```python
from build123d import *

# Parameters (mm, degrees)
ESQUISSE3_R             = 2.5
BOSS_EXTRU_3_DEPTH      = 5
ESQUISSE4_W             = 40
ESQUISSE4_H             = 30
ENL_V_MAT_EXTRU_1_DEPTH = 161.669919512


with BuildPart() as part:
    # Esquisse3 → Boss.-Extru.3 (new body)
    with BuildSketch(Plane(origin=(0, 0, 0), x_dir=(1, 0, 0), z_dir=(0, 1, 0))):
        with BuildLine():
            Line((-115, -25), (-25, -25))
            Line((-25, -25), (-24.99494949, -24.500051021))
            ThreePointArc((-24.99494949, -24.500051021), (-17.805293657, -30.132565736), (-9.403186381, -33.713203436))
            Line((-9.403186381, -33.713203436), (35.849364905, -112.092921435))
            Line((35.849364905, -112.092921435), (79.150635095, -87.092921435))
            Line((79.150635095, -87.092921435), (34.150635095, -9.150635095))
            Line((34.150635095, -9.150635095), (33.715141323, -9.396235714))
            ThreePointArc((33.715141323, -9.396235714), (34.998214236, -0.353553761), (33.898083809, 8.713203436))
            Line((33.898083809, 8.713203436), (79.150635095, 87.092921435))
            Line((79.150635095, 87.092921435), (35.849364905, 112.092921435))
            Line((35.849364905, 112.092921435), (-9.150635095, 34.150635095))
            Line((-9.150635095, 34.150635095), (-8.720191833, 33.896286735))
            ThreePointArc((-8.720191833, 33.896286735), (-17.19292058, 30.486119496), (-24.494897428, 25))
            Line((-24.494897428, 25), (-115, 25))
            Line((-115, 25), (-115, -25))
        make_face()
        with Locations(Location((-110, -20, 0), (0, 0, 270))):
            Circle(ESQUISSE3_R, mode=Mode.SUBTRACT)
        with Locations(Location((-110, 20, 0), (0, 0, 270))):
            Circle(ESQUISSE3_R, mode=Mode.SUBTRACT)
        with Locations(Location((72.320508076, -85.262794416, 0), (0, 0, 270))):
            Circle(ESQUISSE3_R, mode=Mode.SUBTRACT)
        with Locations(Location((37.679491924, -105.262794416, 0), (0, 0, 270))):
            Circle(ESQUISSE3_R, mode=Mode.SUBTRACT)
        with Locations(Location((72.320508076, 85.262794416, 0), (0, 0, 270))):
            Circle(ESQUISSE3_R, mode=Mode.SUBTRACT)
        with Locations(Location((37.679491924, 105.262794416, 0), (0, 0, 270))):
            Circle(ESQUISSE3_R, mode=Mode.SUBTRACT)
    extrude(amount=BOSS_EXTRU_3_DEPTH)

    # Esquisse4 → Enlèv. mat.-Extru.1 (cut, through all)
    with BuildSketch(Plane(origin=(0, 5, 0), x_dir=(1, 0, 0), z_dir=(0, 1, 0))):
        Rectangle(ESQUISSE4_W, ESQUISSE4_H)
    extrude(amount=-ENL_V_MAT_EXTRU_1_DEPTH, mode=Mode.SUBTRACT)


solid = part.part
```
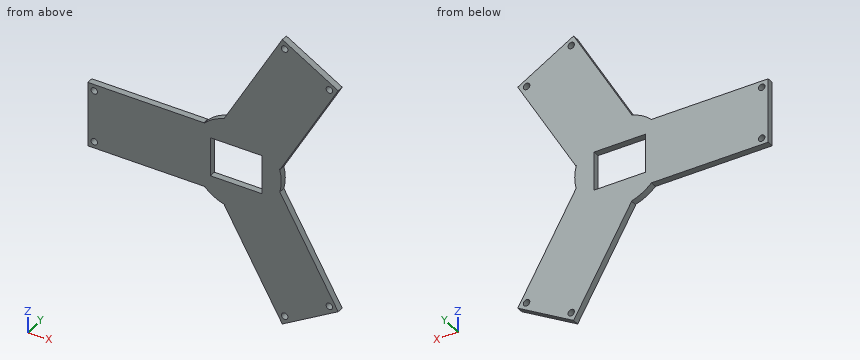
Check sheet for the modelled part. Datum: model origin and axes. Units: mm. Round coordinates to 2 decimals unless told otherwise and drop trailing zeros. Order: outer loops, then holes, each group sorted by start corner. A loop starts at its lowest first (then second) coordinate and runs counter-clockwise, first axis right, second up. Notation, with made-up numbers: (87.25, 77.5) - (140.25, 77.5) arc R13 ccw to (140.25, 100.5) - close; hole circle Ø7 at (26.5, 59). An arc over 180 degrees is marked (long way). Answer as CSV lines item,"result". Start each with the question number.
1) Section check A-A (x = -110). Record the cut outline in (y, z).
2) Section check C-C (x = 65). Record the cut outline in (y, z), then the cut area to 3 significant figures.
3) Section check D-D (z = -20). Record the cut outline in (x, y).
4) Section check B-B (y = 3.2). Record the cut outline in (x, z), then the cut area to 3 significant figures.
5) Scan lines: probe 1 along Z at (x, y) = (60.5, 0.2); probe 2 along Z at (x, y) = (-40.5, 4.1); probe 3 along Z at (x, y) = (62, 1.9). Record each from-to range of solid material in increasing order.
6) Depth check by flat-ended pin: pin 1 (1 mm diameter, centred on x = -85.5, y = 3.5, fed in from +Z); pin 2 (1 mm diameter, centred on y = 4, z = 87, fed in from -X); pin 3 (2.5 mm diameter, centred on y = 2, z = -7, fed in from +X). Enter the tip coordinate at first touch or a pass-through.
Determined:
1,outline,"(0, -25) - (5, -25) - (5, -22.5) - (0, -22.5) - close; (0, -17.5) - (5, -17.5) - (5, 17.5) - (0, 17.5) - close; (0, 22.5) - (5, 22.5) - (5, 25) - (0, 25) - close"
2,outline,"(0, -95.26) - (5, -95.26) - (5, -62.58) - (0, -62.58) - close; (0, 62.58) - (5, 62.58) - (5, 95.26) - (0, 95.26) - close"
2,area,"327 mm^2"
3,outline,"(-115, 0) - (-112.5, 0) - (-112.5, 5) - (-115, 5) - close; (-107.5, 0) - (40.41, 0) - (40.41, 5) - (-107.5, 5) - close"
4,outline,"(-115, -25) - (-24.49, -25) arc R35 ccw to (-8.72, -33.9) - (-9.15, -34.15) - (35.85, -112.09) - (79.15, -87.09) - (33.9, -8.71) arc R35 ccw to (33.72, 9.4) - (34.15, 9.15) - (79.15, 87.09) - (35.85, 112.09) - (-9.4, 33.71) arc R35 ccw to (-24.99, 24.5) - (-25, 25) - (-115, 25) - close; hole circle Ø5 at (-110, -20); hole circle Ø5 at (-110, 20); hole (-20, -15) - (20, -15) - (20, 15) - (-20, 15) - close; hole circle Ø5 at (37.68, -105.26); hole circle Ø5 at (37.68, 105.26); hole circle Ø5 at (72.32, -85.26); hole circle Ø5 at (72.32, 85.26)"
4,area,"15,000 mm^2"
5,probe 1,"-97.86 to -54.79, 54.79 to 97.86"
5,probe 2,"-25 to 25"
5,probe 3,"-96.99 to -57.39, 57.39 to 96.99"
6,pin 1,"z = 25"
6,pin 2,"x = 21.07"
6,pin 3,"x = 34.52"
